The figure shows three views and two pictorial views of one solid part (mm, origin at its lowest corner). Answer the questions. Coordinates: 2 decimals unless noted, no trailing zeros. Loops run counter-clockwise (first coordinate to the right, second up) from the corner with the lowest first, then second, coordinate; pieces in that order, holes last.
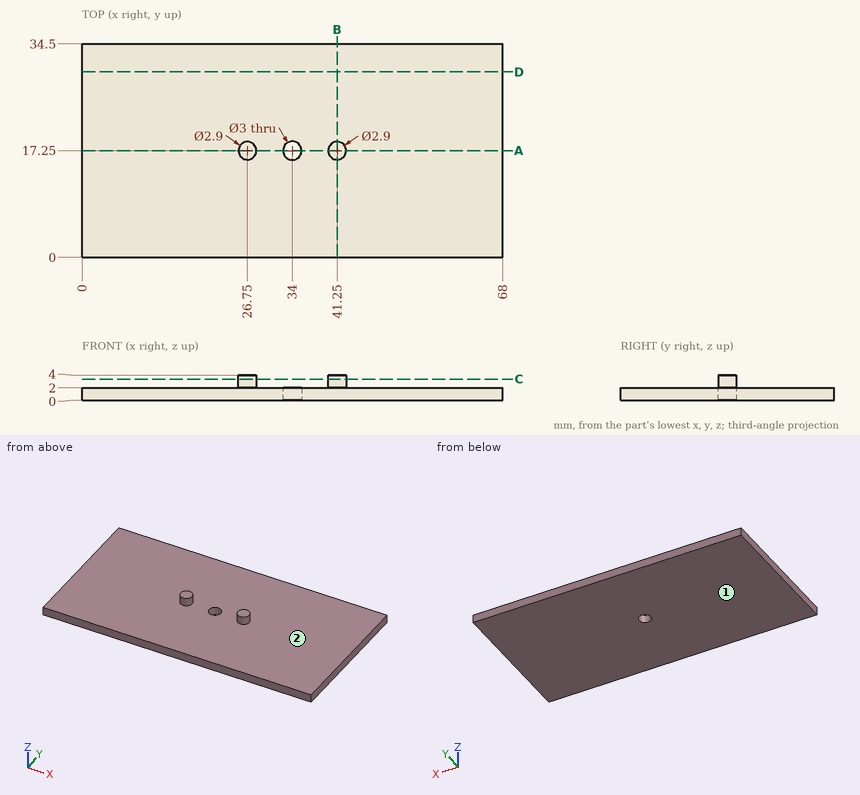
Q1. A cutting plane is placed at A-A (y = 17.25). Give the vertices of the cut face in (x, z).
Findings below:
outline: (0, 0) - (32.5, 0) - (32.5, 2) - (28.2, 2) - (28.2, 4) - (25.3, 4) - (25.3, 2) - (0, 2) - close; (35.5, 0) - (68, 0) - (68, 2) - (42.7, 2) - (42.7, 4) - (39.8, 4) - (39.8, 2) - (35.5, 2) - close
Q2. A cutting plane is placed at C-C (z = 3.4). Give the vertices of the cut face in (x, y), then the cut area to 3 significant figures.
Findings below:
outline: circle Ø2.9 at (26.75, 17.25); circle Ø2.9 at (41.25, 17.25)
area: 13.2 mm2
Q3. A cutting plane is placed at B-B (x = 41.25). Give the vertices of the cut face in (y, z), then the cut area to 3 significant figures.
Findings below:
outline: (0, 0) - (34.5, 0) - (34.5, 2) - (18.7, 2) - (18.7, 4) - (15.8, 4) - (15.8, 2) - (0, 2) - close
area: 74.8 mm2
Q4. Determine the mould class of the marked faces 1 and 2 for opening direction Z: +Z half, -Z half, draft (parallel to the pull), parting line (faces both ways), or undercut.
Findings below:
face 1: -Z half
face 2: +Z half
Q5. Flat-ended cylindrical pins translate along their axes: pin 1 Ø1.8 at (x, y) = (34, 17.25) entering from +Z; pin 2 Ø3 at (x, y) = (11, 25.5) entering from +Z. Find the tip coordinate at first contact, or state that the pin passes through.
Findings below:
pin 1: passes through
pin 2: stops at z = 2
Q6. Straight lines are drawn through the part: probe 1 along Y at (x, z) = (34, 1.5); probe 2 along Z at (x, y) = (38.5, 26); probe 3 along X at (y, z) = (17, 2.6). For each, find the intervals that lie inside material, in ascending order.
Findings below:
probe 1: y = 0 to 15.75, 18.75 to 34.5
probe 2: z = 0 to 2
probe 3: x = 25.32 to 28.18, 39.82 to 42.68
Q7. A cutting plane is placed at D-D (y = 30). Give the vertices of the cut face in (x, z).
Findings below:
outline: (0, 0) - (68, 0) - (68, 2) - (0, 2) - close
